Build history of the part. All positions in model axes, mm. Face numbers are marked on the shaded views. A direction names the side the tool comes from. Coordinates: 2 decimals unless noted, no trailing zeros. Loops run counter-clockwise (first coordinate to the right, second up) from the corner with the lowest first, then second, coordinate; pieces in that order, holes last.
Item 1: Drill centre lines: line 1 along X through (y, z) = (-2.2, 16.25); line 2 along Z through (x, y) = (15.5, -3.75); line 3 along Z through (x, y) = (15, -4.5). Where is each one in solid material? Low to high.
Item 2: Cut at B-B (z = 17.5). List the corners of the cut face in (x, y), and give its area (3 significant figures).
Item 3: Mould opens along Z. For the marked faces 1, 2 and 3 say: released by +Z, released by -Z, zero draft, split by the parting line, or undercut.
Item 4: Cut at C-C (x = 6). List the corners of the cut face in (y, z), and give its area (3 significant figures).
Item 5: 3-axis set-ups, long thin cutter, end or side, ignore diameter. For the marked faces 4 and 5: which of +Z, -Z, +X, -X, +Y, -Y reach the whole face in a straight line?
Item 6: Flat gauge pins, fed straight in: pin 1 (6 mm diameter, centred on x = -8, z = 20.5, fed in from +Y); pin 2 (2.5 mm diameter, centred on x = -0.5, y = -2.5, fed in from +Z); pin 3 (2 mm diameter, centred on y = -2.5, z = 23, fed in from -X). Where does each tip first touch, or does it go through?
Item 7: Cut at D-D (z = 27). List the corners of the cut face in (x, y), and give its area (3 significant figures).
Item 8: Cut at A-A (y = -2.35). List the corners of the cut face in (x, z).
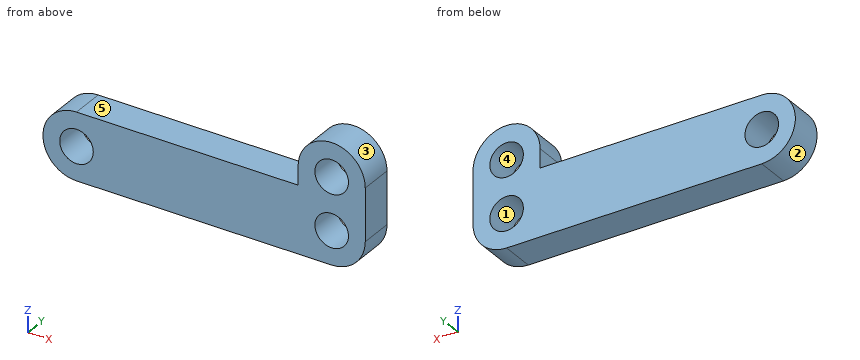
from build123d import *

# Parameters (mm, degrees)
F0_R     = 2.5
F1_DEPTH = 5


with BuildPart() as f1:
    # F0 (on Front) → F1 (new body)
    with BuildSketch(Plane.XZ):
        with BuildLine():
            Line((10.71558, 21.128206), (-22.28442, 21.128206))
            ThreePointArc((-22.28442, 21.128206), (-27.28442, 16.128206), (-22.28442, 11.128206))
            Line((-22.28442, 11.128206), (15.71558, 11.128206))
            ThreePointArc((15.71558, 11.128206), (19.251113, 12.592672), (20.71558, 16.128206))
            Line((20.71558, 16.128206), (20.71558, 23.928206))
            ThreePointArc((20.71558, 23.928206), (15.71558, 28.928206), (10.71558, 23.928206))
            Line((10.71558, 23.928206), (10.71558, 21.128206))
        make_face()
        with Locations((-22.28442, 16.128206)):
            Circle(F0_R, mode=Mode.SUBTRACT)
        with Locations((15.71558, 16.128206)):
            Circle(F0_R, mode=Mode.SUBTRACT)
        with Locations((15.71558, 23.928206)):
            Circle(F0_R, mode=Mode.SUBTRACT)
    extrude(amount=F1_DEPTH)


solid = f1.part
Filled sheet:
1. line 1: x = -27.28 to -24.78, -19.79 to 13.22, 18.21 to 20.72
1. line 2: z = 11.13 to 13.64, 18.62 to 21.44, 26.42 to 28.92
1. line 3: z = 11.13 to 13.73, 18.52 to 21.53, 26.32 to 28.88
2. outline: (-27.09, -5) - (-24.37, -5) - (-24.37, 0) - (-27.09, 0) - close; (-20.19, -5) - (13.63, -5) - (13.63, 0) - (-20.19, 0) - close; (17.81, -5) - (20.72, -5) - (20.72, 0) - (17.81, 0) - close
2. area: 197 mm2
3. face 1: undercut
3. face 2: split by the parting line
3. face 3: released by +Z
4. outline: (-5, 11.13) - (0, 11.13) - (0, 21.13) - (-5, 21.13) - close
4. area: 50.0 mm2
5. face 4: +Y, -Y
5. face 5: +Z, -X, +Y, -Y
6. pin 1: stops at y = 0
6. pin 2: stops at z = 21.13
6. pin 3: stops at x = 10.72
7. outline: (11.77, -5) - (19.66, -5) - (19.66, 0) - (11.77, 0) - close
7. area: 39.5 mm2
8. outline: (-22.28, 11.13) - (15.72, 11.13) arc R5 ccw to (20.72, 16.13) - (20.72, 23.93) arc R5 ccw to (10.72, 23.93) - (10.72, 21.13) - (-22.28, 21.13) arc R5 ccw to start; hole circle Ø5 at (-22.28, 16.13); hole circle Ø5 at (15.72, 16.13); hole circle Ø5 at (15.72, 23.93)
